```python
from build123d import *

# Parameters (mm, degrees)
F0_W     = 350
F0_H     = 100
F1_DEPTH = 10
F2_SIZE2 = 19.99999
F2_SIZE  = 19.99999
F3_SIZE2 = 19.99999
F3_SIZE  = 19.99999


# Not quite as in the source:
# - a fillet or chamfer is up to 0.001 mm smaller than in the source, because OpenCascade refuses the exact size


with BuildPart() as f1:
    # F0 (on Front) → F1 (new body, symmetric)
    with BuildSketch(Plane.XZ):
        with Locations((175, 50)):
            Rectangle(F0_W, F0_H)
    extrude(amount=F1_DEPTH, both=True)

    # F2 (size 20 and 20 in the source; OpenCascade refuses exactly that, so slightly less here)
    f2_edges = [f1.edges().sort_by_distance(p)[0] for p in [
        (0, -10, 50),
    ]]
    chamfer(f2_edges, length=F2_SIZE, length2=F2_SIZE2)

    # F3 (size 20 and 20 in the source; OpenCascade refuses exactly that, so slightly less here)
    f3_edges = [f1.edges().sort_by_distance(p)[0] for p in [
        (350, -10, 50),
    ]]
    chamfer(f3_edges, length=F3_SIZE, length2=F3_SIZE2)


solid = f1.part
```
Here's how the part is built. I have some questions about the finished solid (model axes, mm). Give positions to 0.01 mm unless a question says otherwise; leave off trailing zeros. Write each loop counter-clockwise with the first axis right and the second up, starting at its lowest first coordinate (ties: lowest second). Pieces come first, ordered by that corner, then holes. Notation, with made-up numbers: M 15.5,-6.5 L 45.5,-6.5 A18 ccw 45.5,19.5 Z; hole C 44,7 d3. An arc over 180 degrees is marked long. Put each result on its own line as item: value. Start each with the question number.
Item 1: If we section it at A-A, the plane y = 3: Write out the boundary of the cut face in (x, z), then the cut area to 3 significant figures.
Item 2: I need wall thicknesses on L1, parallel to X at y = -1, z = 65; L2, parallel to X at y = 0.5, z = 34.5; L3, parallel to Y at x = 14, z = 79. Which ranges of each line are inside material? Lowest first, please. Write a range as from..to.
Item 3: Will these pins go through, and if not, where does the flat tip stop? pin 1 (8 mm diameter, centred on y = -2, z = 27.5, fed in from -X); pin 2 (4 mm diameter, centred on y = 7.5, z = 29.5, fed in from -X); pin 3 (12 mm diameter, centred on y = -1.5, z = 27.5, fed in from +X).
Values:
1. outline: M 7,0 L 343,0 L 343,100 L 7,100 Z
1. area: 33,600 mm²
2. L1: 11..339
2. L2: 9.5..340.5
2. L3: -4..10
3. pin 1: x = 8
3. pin 2: x = 0.5
3. pin 3: x = 344.5
